Verification items for the finished model (mm, model axes). A direction names the side the tool comes from. Give positions to 0.01 mm unless a question says otherwise; leave off trailing zeros. Write each loop counter-clockwise with the first axis right and the second up, starting at its lowest first coordinate (ties: lowest second). Pieces come first, ordered by that corner, then holes. Notation, with made-up numbers: (-25, 29) -> (-10, 29) arc R20 ccw to (-10, 43) -> close; hole circle Ø4 at (76.5, -1.75). An arc over 180 degrees is marked (long way). Write item = value, one per line.
Autodesk Inventor part; units mm, degrees
ref_plane "YZ Plane" through (0, 0, 0) normal (1, 0, 0) x (0, 1, 0)
ref_plane "XZ Plane" through (0, 0, 0) normal (0, 1, 0) x (-1, 0, 0)
ref_plane "XY Plane" through (0, 0, 0) normal (0, 0, 1) x (1, 0, 0)
sketch "Sketch1" plane through (0, 0, 0) normal (0, 0, 1) x (1, 0, 0)
  line L0 (-10, 0) -> (-38, 0)
  line L1 (-38, 0) -> (-38, 60)
  arc A0 (0, 10) -> (-10, 0) centre (0, 0) ccw
  line L2 (0, 10) -> (0, 100)
  line L3 (0, 100) -> (-15, 100)
  line L4 (-15, 100) -> (-15, 80)
  line L5 (0, 10) -> (0, 0)
  line L6 (-38, 60) -> (-15, 80)
  dimension "d5" = 60
  dimension "d9" = 20
  dimension "d11" = 15
  dimension "d12" = 20
revolve "Revolution1" add sketch "Sketch1" angle 360 about axis through (0, 10, 0) along (0, 1, 0)
fillet "Fillet1" radius 10 1 edges at (15, 80, 0)
fillet "Fillet1" radius 20 1 edges at (38, 60, 0)
fillet "Fillet3" radius 10 1 edges at (10, 0, 0)
shell "Shell1" thickness 1 removed faces 1 at (4.4273, 100, -2.3236)
sketch "Sketch2" plane through (0, 0, 0) normal (1, 0, 0) x (0, 1, 0)
  line L0 (100, -15) -> (100, 15)
  line L1 (100, 0) -> (90, 0)
  circle A0 centre (90, 0) radius 3.5
  point P0 (0, 0)
  dimension "d20" = 10
  dimension "d21" = 7
extrude "Extrusion1" cut sketch "Sketch2" along normal mid plane 50
sketch "Sketch3" plane through (0, 0, 0) normal (0, -1, 0) x (1, 0, 0)
  circle A0 centre (0, 0) radius 37
  circle A1 centre (0, 0) radius 38
  circle A2 centre (0, 0) radius 39
  dimension "d24" = 76
  dimension "d25" = 78
extrude "Extrusion2" add sketch "Sketch3" against normal blind 220 contours A2
properties part number "1"
Item 1: Sectioned sample at A-A on y = 90. Record the cut outline in (x, z), then the cut area to 3 significant figures.
Response values:
outline = circle Ø78 at (0, 0); (-14.59, -3.5) arc R15 ccw to (14.59, -3.5) -> (13.56, -3.5) arc R14 cw to (-13.56, -3.5) -> close; (-14.59, 3.5) -> (-13.56, 3.5) arc R14 cw to (13.56, 3.5) -> (14.59, 3.5) arc R15 ccw to start; hole circle Ø76 at (0, 0)
area = 319 mm^2
Item 2: Sectioned sample at D-D on y = 184. Record the cut outline in (x, z), then the cut area to 3 significant figures.
Response values:
outline = circle Ø78 at (0, 0); hole circle Ø76 at (0, 0)
area = 242 mm^2
Item 3: Sectioned sample at B-B on z = 0. Give the number of separate pieces and of enclosed holes in the cut face, then the cut area to 3 significant figures.
Response values:
separate_pieces = 3
enclosed_holes = 0
area = 725 mm^2
Item 4: Mould release check, pull along Z, two halves, no side actions. Record for faces 4 (the flat face through (17, 0, -8)), 5 (the cylindrical face through (14.268, 93.233, 1.341)), 6 (the cylindrical face through (-5.077, 108.46, 38.668)): +Z half, -Z half, draft (parallel to the pull), parting line (faces both ways), or undercut.
Response values:
face_4 = draft
face_5 = undercut
face_6 = parting line
Item 5: Material ranges on line 1 (Z direction, x = 0, y = 88); line 2 (Z direction, x = 0, y = 23); line 3 (X direction, y = 92, z = 4.5), recorded low to high.
Response values:
line_1 = -39 to -38, -15 to -14, 14 to 15, 38 to 39
line_2 = -39 to -37, 37 to 39
line_3 = -38.74 to -37.73, -14.31 to -13.26, 13.26 to 14.31, 37.73 to 38.74
Item 6: Set-up check for faces 1 (the cylindrical face through (-12.932, 92.17, 5.362)), 2 (the conical face through (4, 75.6, 18.1)), 3 (the flat face through (8.5, 220, -37.4)): record each of +Z, -Z, +X, -X, +Y, -Y from which the full face is reachable in a straight line by a thin tool's end or side.
Response values:
face_1 = +Y
face_2 = none
face_3 = +Z, -Z, +X, -X, +Y
Item 7: Sectioned sample at C-C on y = 27. Record the cut outline in (x, z), then the cut area to 3 significant figures.
Response values:
outline = circle Ø78 at (0, 0); hole circle Ø74 at (0, 0)
area = 478 mm^2
Item 8: Go/stop test with flat-tipped pins: P1, Ø5, axis at y = 49.5, z = 16.5, coming from the -X side; P2, Ø3, axis at x = 16, y = 121.5, coming from the -Z side; P3, Ø4, axis at x = 28, y = 110.5, coming from the -Z side. Record where each tip stops, or that it passes through.
Response values:
P1 = -36.4
P2 = -36.2
P3 = -29.07
